```python
from build123d import *

# Parameters (mm, degrees)
CUT_EXTRUDE1_DEPTH  = 43.303774347
CIRPATTERN1_COUNT   = 4
SKETCH8_R           = 9.2075
BOSS_EXTRUDE1_DEPTH = 3.175
CUT_EXTRUDE2_DEPTH  = 2.032
SKETCH7_R           = 2.413
CUT_EXTRUDE3_DEPTH  = 43.782415184
FILLET1_R           = 1.27


with BuildPart() as part:
    # Sketch1 → Revolve1 (revolve)
    with BuildSketch(Plane(origin=(0, 0, 0), x_dir=(0, 0, -1), z_dir=(1, 0, 0)), mode=Mode.PRIVATE) as revolve1_sk:
        with BuildLine():
            Line((0, -1.651), (0, 1.651))
            Line((0, 1.651), (0, 2.413))
            Line((0, 2.413), (-29.718, 2.413))
            Line((-29.718, 2.413), (-29.718, 1.651))
            ThreePointArc((-29.718, 1.651), (-28.067, 0), (-29.718, -1.651))
            Line((-29.718, -1.651), (-29.718, -2.413))
            Line((-29.718, -2.413), (0, -2.413))
            Line((0, -2.413), (0, -1.651))
        make_face()
    revolve(revolve1_sk.sketch.rotate(Axis((0, -1.651, 0), (0, 1, 0)), 180), axis=Axis((0, -1.651, 0), (0, 1, 0)))

    # Sketch4 → Cut-Extrude1 (cut, through all)
    with BuildSketch(Plane(origin=(0, 2.413, 0), x_dir=(1, 0, 0), z_dir=(0, 1, 0))):
        with BuildLine():
            Line((-18.150933962, -3.200499383), (-13.725620051, -2.420197142))
            ThreePointArc((-13.725620051, -2.420197142), (-11.215481947, -2.795189817), (-9.436261178, -4.605103146))
            ThreePointArc((-9.436261178, -4.605103146), (-7.424621202, -7.424621202), (-4.605103146, -9.436261178))
            ThreePointArc((-4.605103146, -9.436261178), (-2.795189817, -11.215481947), (-2.420197142, -13.725620051))
            Line((-2.420197142, -13.725620051), (-3.200499383, -18.150933962))
            ThreePointArc((-3.200499383, -18.150933962), (-5.207970247, -20.958954952), (-8.653989227, -21.158640563))
            ThreePointArc((-8.653989227, -21.158640563), (-16.164461018, -16.164461018), (-21.158640563, -8.653989227))
            ThreePointArc((-21.158640563, -8.653989227), (-20.958954952, -5.207970247), (-18.150933962, -3.200499383))
        make_face()
    cut_extrude1 = extrude(amount=-CUT_EXTRUDE1_DEPTH, mode=Mode.SUBTRACT)

    # CirPattern1: Cut-Extrude1 ×4 about axis
    cirpattern1_axis = Axis((0, 0, 0), (0, 1, 0))
    for i in range(1, CIRPATTERN1_COUNT):
        add(cut_extrude1.rotate(cirpattern1_axis, i * 360 / CIRPATTERN1_COUNT), mode=Mode.SUBTRACT)

    # Sketch8 → Boss-Extrude1 (add)
    with BuildSketch(Plane(origin=(0, 2.413, 0), x_dir=(1, 0, 0), z_dir=(0, 1, 0))):
        with Locations(Location((0, 0, 0), (0, 0, 90))):
            Circle(SKETCH8_R)
    extrude(amount=BOSS_EXTRUDE1_DEPTH)

    # Sketch6 → Cut-Extrude2 (cut)
    with BuildSketch(Plane(origin=(0, 5.588, 0), x_dir=(1, 0, 0), z_dir=(0, 1, 0))):
        Polygon((0, 7.112377966), (-6.1595, 3.556188983), (-6.1595, -3.556188983), (0, -7.112377966), (6.1595, -3.556188983), (6.1595, 3.556188983), align=None)
    extrude(amount=-CUT_EXTRUDE2_DEPTH, mode=Mode.SUBTRACT)

    # Sketch7 → Cut-Extrude3 (cut, through all)
    with BuildSketch(Plane(origin=(0, 5.588, 0), x_dir=(1, 0, 0), z_dir=(0, 1, 0))):
        with Locations(Location((0, 0, 0), (0, 0, 270))):
            Circle(SKETCH7_R)
    extrude(amount=-CUT_EXTRUDE3_DEPTH, mode=Mode.SUBTRACT)

    # Fillet1
    fillet1_edges = [part.edges().sort_by_distance(p)[0] for p in [
        (0, 2.413, 9.2075),
    ]]
    fillet(fillet1_edges, radius=FILLET1_R)


solid = part.part
```
Work out the finished part from the listing and answer in its coordinate system (mm). A direction names the side the tool comes from. Give positions to 0.01 mm unless a question says otherwise; leave off trailing zeros. Order: outer loops, then holes, each group sorted by start corner. A loop starts at its lowest first (then second) coordinate and runs counter-clockwise, first axis right, second up. Notation, with made-up numbers: (37, 45) - (88, 45) arc R20 cw to (88, 53) - close; hole circle Ø3 at (29.25, 68.5). An arc over 180 degrees is marked (long way). One line per item, written item: value. Start each with the question number.
1. Which of the six approach directions +Z, -Z, +X, -X, +Y, -Y give full straight-line access (tool end or side, diameter ignored) to faces 4 (the face through (20.98, 0.03, -5.25)), 5 (the face through (-3.037, 4.586, -5.359))?
2. Consider line 1 (X direction, y = 1.75, z = 13); line 2 (X direction, y = 1.25, z = 8); line 3 (Z direction, x = 11, y = 1). Determine where each line is inside the solid, lowest interval first.
3. Section A-A, the plane z = 0 is taken. Write down the section's boundary in (x, y), then the cut area to 3 significant figures.
4. Section B-B, the plane y = 0.25 is taken. Count the separate pieces of the cut face and the enclosed holes in it, then the cut area to 3 significant figures.
5. Each of these flat-tipped pins is pushed along its axis until it touches: pin 1 Ø1.5 at (y, z) = (0, -0.5) entering from +X; pin 2 Ø0.6 at (y, z) = (4.5, 1) entering from +X; pin 3 Ø0.6 at (y, z) = (4.5, 1.5) entering from -X; pin 4 Ø6 at (x, z) = (8.5, 11.5) entering from +Y. Where does it stop, or does it pass through?
6. For a pull along X with two mould halves and no side action, classify faces 1 (the face through (-2.2, 5.588, 6.3)), 2 (the face through (-8.926, 2.027, -28.346)), 3 (the face through (-2.816, 0.034, -15.969)) as released by +X, released by -X, zero draft, split by the parting line, or undercut.
Filled sheet:
1. face 4: +Y, -Y
1. face 5: +Y
2. line 1: -26.72 to -18.8, -2.36 to 2.36, 18.8 to 26.72
2. line 2: -27.5 to -21.36, -6.8 to 6.8, 21.36 to 27.5
2. line 3: -26.19 to -20.04, -2.91 to 2.91, 20.04 to 26.19
3. outline: (-29.72, -2.41) - (-2.41, -2.41) - (-2.41, 3.56) - (-6.16, 3.56) - (-6.16, 5.59) - (-9.21, 5.59) - (-9.21, 3.68) arc R1.27 cw to (-10.48, 2.41) - (-29.72, 2.41) - (-29.72, 1.65) arc R1.65 cw to (-29.72, -1.65) - close; (2.41, -2.41) - (29.72, -2.41) - (29.72, -1.65) arc R1.65 cw to (29.72, 1.65) - (29.72, 2.41) - (10.48, 2.41) arc R1.27 cw to (9.21, 3.68) - (9.21, 5.59) - (6.16, 5.59) - (6.16, 3.56) - (2.41, 3.56) - close
3. area: 284 mm²
4. separate pieces: 1
4. enclosed holes: 5
4. area: 1,510 mm²
5. pin 1: x = 28.24
5. pin 2: x = 9.18
5. pin 3: x = -9.13
5. pin 4: through
6. face 1: zero draft
6. face 2: split by the parting line
6. face 3: undercut
